Geometry: see drawing. Coordinates: mm, zero at the bounding-box minimum. Round coordinates to 2 decimals unless told otherwise and drop trailing zeros. Write each loop counter-clockwise with the first axis right and the second up, starting at its lowest first coordinate (ties: lowest second). Pieces come first, ordered by that corner, then holes. Notation, with made-up numbers: M 65.5,59 L 117.5,59 A26 ccw 117.5,84 Z; hole C 69.25,49.25 d6. An arc over 180 degrees is marked long. Use one line per item in the form item = value. Start each with the question number.
Item 1: Section query A-A (z = 1.95). Return loops of the section in (x, y), and give its area (3 significant figures).
Item 2: Pin query (flat end, axial travel): pin 1 Ø2.5 at (x, z) = (45.5, 1.5) entering from +Y; pin 2 Ø3 at (x, z) = (53.5, 3) entering from -Y. Return the tip coordinate at first contact, or that it passes through.
Item 3: Section query B-B (x = 49). Return loops of the section in (y, z), and give its area (3 significant figures).
Item 4: Ray query, probe 1 along Y at (x, z) = (61, 0.75). Return the intervals inside material, ascending.
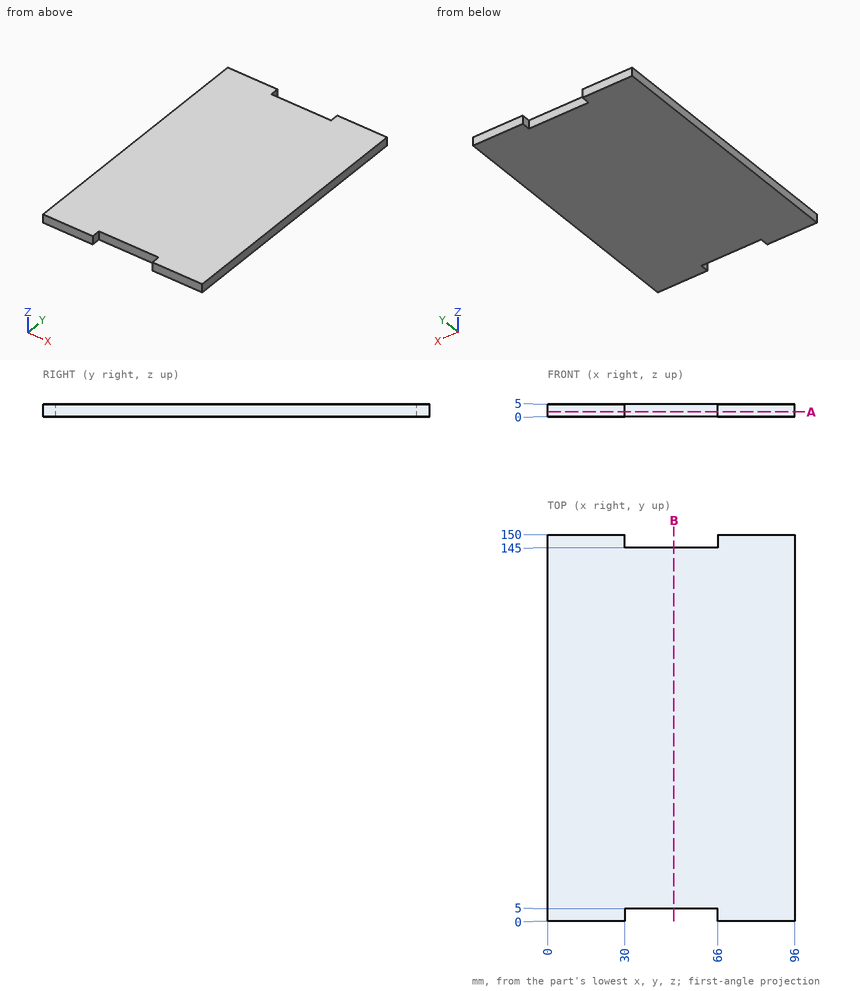
Working result:
q1.outline = M 0,0 L 30,0 L 30,5 L 66,5 L 66,0 L 96,0 L 96,150 L 66,150 L 66,145 L 30,145 L 30,150 L 0,150 Z
q1.area = 14,000 mm²
q2.pin_1 = 145
q2.pin_2 = 5
q3.outline = M 5,0 L 145,0 L 145,5 L 5,5 Z
q3.area = 700 mm²
q4.probe_1 = 5 to 145
